from build123d import *

# Parameters (mm, degrees)
F2_DEPTH  = 3.175
F4_DEPTH  = 3.175
F5_R      = 0.8001
F6_DEPTH  = 3.2004
F7_R      = 0.8001
F8_DEPTH  = 25.4
F9_W      = 5.7083697757
F9_H      = 1.5914540656
F10_DEPTH = 3.175
F12_DEPTH = 25.4
F13_R     = 0.3937
F14_DEPTH = 25.4


with BuildPart() as f2:
    # F1 (on face) → F2 (new body)
    with BuildSketch(Plane.XY):
        with BuildLine():
            ThreePointArc((-1.5819782441, 9.3927083333), (-6.1504992572, -7.2730312723), (9.525, 0))
            ThreePointArc((9.525, 0), (7.2730312723, 6.1504992572), (1.5819782441, 9.3927083333))
            ThreePointArc((1.5819782441, 9.3927083333), (1.191708121, 9.4501564407), (0.7993940003, 9.4913958))
            ThreePointArc((0.7993940003, 9.4913958), (0, 8.7249), (-0.7993940003, 9.4913958))
            ThreePointArc((-0.7993940003, 9.4913958), (-1.191708121, 9.4501564407), (-1.5819782441, 9.3927083333))
        make_face()
        with BuildLine():
            ThreePointArc((0.7993940003, 9.4913958), (1.191708121, 9.4501564407), (1.5819782441, 9.3927083333))
            ThreePointArc((1.5819782441, 9.3927083333), (0, 11.1125), (-1.5819782441, 9.3927083333))
            ThreePointArc((-1.5819782441, 9.3927083333), (-1.191708121, 9.4501564407), (-0.7993940003, 9.4913958))
            ThreePointArc((-0.7993940003, 9.4913958), (-0.0168058077, 10.3249234806), (0.8001, 9.525))
            ThreePointArc((0.8001, 9.525), (0.7999234806, 9.5081941923), (0.7993940003, 9.4913958))
        make_face()
    extrude(amount=F2_DEPTH)

    # F3 (on Top) → F4 (join)
    with BuildSketch(Plane.XY):
        with BuildLine():
            ThreePointArc((0.7993940003, 9.4913958), (1.191708121, 9.4501564407), (1.5819782441, 9.3927083333))
            ThreePointArc((1.5819782441, 9.3927083333), (0, 11.1125), (-1.5819782441, 9.3927083333))
            ThreePointArc((-1.5819782441, 9.3927083333), (-1.191708121, 9.4501564407), (-0.7993940003, 9.4913958))
            ThreePointArc((-0.7993940003, 9.4913958), (-0.0168058077, 10.3249234806), (0.8001, 9.525))
            ThreePointArc((0.8001, 9.525), (0.7999234806, 9.5081941923), (0.7993940003, 9.4913958))
        make_face()
        with BuildLine():
            ThreePointArc((-0.7993940003, 9.4913958), (0, 9.525), (0.7993940003, 9.4913958))
            ThreePointArc((0.7993940003, 9.4913958), (0.7999234806, 9.5081941923), (0.8001, 9.525))
            ThreePointArc((0.8001, 9.525), (-0.0168058077, 10.3249234806), (-0.7993940003, 9.4913958))
        make_face()
        with BuildLine():
            ThreePointArc((4.2410481532, -8.5287241462), (6.5317636161, -8.99020135), (6.8007427217, -6.6689971835))
            ThreePointArc((6.8007427217, -6.6689971835), (6.51877471, -6.9448687015), (6.2256258064, -7.2088284984))
            ThreePointArc((6.2256258064, -7.2088284984), (6.3542336867, -7.4427136488), (6.3987545281, -7.7058868714))
            ThreePointArc((6.3987545281, -7.7058868714), (5.8298612048, -8.4718525904), (4.9321791435, -8.1485725067))
            ThreePointArc((4.9321791435, -8.1485725067), (4.5905504655, -8.3458056186), (4.2410481532, -8.5287241462))
        make_face()
        with BuildLine():
            ThreePointArc((4.9321791435, -8.1485725067), (5.5986545281, -7.7058868714), (6.2256258064, -7.2088284984))
            ThreePointArc((6.2256258064, -7.2088284984), (5.1283675477, -7.0585923742), (4.9321791435, -8.1485725067))
        make_face()
        with BuildLine():
            ThreePointArc((9.4218546282, 1.3979557805), (10.5686155373, 3.43395135), (8.4441383039, 4.4070572159))
            ThreePointArc((8.4441383039, 4.4070572159), (8.6193748012, 4.0536407137), (8.779827493, 3.6932714756))
            ThreePointArc((8.779827493, 3.6932714756), (9.5154003585, 3.6004167674), (9.8589133177, 2.9433868714))
            ThreePointArc((9.8589133177, 2.9433868714), (9.6960868018, 2.4596074625), (9.2738801556, 2.1727337295))
            ThreePointArc((9.2738801556, 2.1727337295), (9.3558909247, 1.7868771657), (9.4218546282, 1.3979557805))
        make_face()
        with BuildLine():
            ThreePointArc((9.2738801556, 2.1727337295), (9.0588133177, 2.9433868714), (8.779827493, 3.6932714756))
            ThreePointArc((8.779827493, 3.6932714756), (8.297872999, 2.6961423742), (9.2738801556, 2.1727337295))
        make_face()
        with BuildLine():
            ThreePointArc((-8.2587133177, 2.9433868714), (-8.4017834218, 3.3999739122), (-8.779827493, 3.6932714756))
            ThreePointArc((-8.779827493, 3.6932714756), (-9.0588133177, 2.9433868714), (-9.2738801556, 2.1727337295))
            ThreePointArc((-9.2738801556, 2.1727337295), (-8.5750339088, 2.3061133873), (-8.2587133177, 2.9433868714))
        make_face()
        with BuildLine():
            ThreePointArc((-6.2256258064, -7.2088284984), (-6.51877471, -6.9448687015), (-6.8007427217, -6.6689971835))
            ThreePointArc((-6.8007427217, -6.6689971835), (-6.5317636161, -8.99020135), (-4.2410481532, -8.5287241462))
            ThreePointArc((-4.2410481532, -8.5287241462), (-4.5905504655, -8.3458056186), (-4.9321791435, -8.1485725067))
            ThreePointArc((-4.9321791435, -8.1485725067), (-6.0689415084, -8.3531813686), (-6.2256258064, -7.2088284984))
        make_face()
        with BuildLine():
            ThreePointArc((-4.7985545281, -7.7058868714), (-5.3354813054, -6.9503077128), (-6.2256258064, -7.2088284984))
            ThreePointArc((-6.2256258064, -7.2088284984), (-5.5986545281, -7.7058868714), (-4.9321791435, -8.1485725067))
            ThreePointArc((-4.9321791435, -8.1485725067), (-4.8326888091, -7.9370935482), (-4.7985545281, -7.7058868714))
        make_face()
        with BuildLine():
            ThreePointArc((-0.7993940003, 9.4913958), (0, 8.7249), (0.7993940003, 9.4913958))
            ThreePointArc((0.7993940003, 9.4913958), (0, 9.525), (-0.7993940003, 9.4913958))
        make_face()
        with BuildLine():
            ThreePointArc((6.3987545281, -7.7058868714), (6.3542336867, -7.4427136488), (6.2256258064, -7.2088284984))
            ThreePointArc((6.2256258064, -7.2088284984), (5.5986545281, -7.7058868714), (4.9321791435, -8.1485725067))
            ThreePointArc((4.9321791435, -8.1485725067), (5.8298612048, -8.4718525904), (6.3987545281, -7.7058868714))
        make_face()
        with BuildLine():
            ThreePointArc((9.8589133177, 2.9433868714), (9.5154003585, 3.6004167674), (8.779827493, 3.6932714756))
            ThreePointArc((8.779827493, 3.6932714756), (9.0588133177, 2.9433868714), (9.2738801556, 2.1727337295))
            ThreePointArc((9.2738801556, 2.1727337295), (9.6960868018, 2.4596074625), (9.8589133177, 2.9433868714))
        make_face()
        with BuildLine():
            ThreePointArc((-9.2738801556, 2.1727337295), (-9.0588133177, 2.9433868714), (-8.779827493, 3.6932714756))
            ThreePointArc((-8.779827493, 3.6932714756), (-9.8197536364, 3.1906313686), (-9.2738801556, 2.1727337295))
        make_face()
        with BuildLine():
            ThreePointArc((-4.9321791435, -8.1485725067), (-5.5986545281, -7.7058868714), (-6.2256258064, -7.2088284984))
            ThreePointArc((-6.2256258064, -7.2088284984), (-6.0689415084, -8.3531813686), (-4.9321791435, -8.1485725067))
        make_face()
        with BuildLine():
            ThreePointArc((-8.779827493, 3.6932714756), (-8.6193748012, 4.0536407137), (-8.4441383039, 4.4070572159))
            ThreePointArc((-8.4441383039, 4.4070572159), (-10.5686155373, 3.43395135), (-9.4218546282, 1.3979557805))
            ThreePointArc((-9.4218546282, 1.3979557805), (-9.3558909247, 1.7868771657), (-9.2738801556, 2.1727337295))
            ThreePointArc((-9.2738801556, 2.1727337295), (-9.8197536364, 3.1906313686), (-8.779827493, 3.6932714756))
        make_face()
    extrude(amount=F4_DEPTH)

    # F5 (on face) → F6 (cut)
    with BuildSketch(Plane.XY.offset(3.175)):
        with Locations((0, 9.525)):
            Circle(F5_R)
        with Locations((-9.0588133177, 2.9433868714)):
            Circle(F5_R)
        with Locations((-5.5986545281, -7.7058868714)):
            Circle(F5_R)
        with Locations((5.5986545281, -7.7058868714)):
            Circle(F5_R)
        with Locations((9.0588133177, 2.9433868714)):
            Circle(F5_R)
    extrude(amount=-F6_DEPTH, mode=Mode.SUBTRACT)

    # F7 (on face) → F8 (cut)
    with BuildSketch(Plane.XY.offset(3.175)):
        with BuildLine():
            ThreePointArc((6.8007427217, -6.6689971835), (8.8176725791, -3.6019821332), (9.525, 0))
            Line((9.525, 0), (0, 0))
            Line((0, 0), (0, -9.525))
            ThreePointArc((0, -9.525), (2.1782478632, -9.2725865456), (4.2410481532, -8.5287241462))
            ThreePointArc((4.2410481532, -8.5287241462), (6.5317636161, -8.99020135), (6.8007427217, -6.6689971835))
        make_face()
        with Locations((5.5986545281, -7.7058868714)):
            Circle(F7_R, mode=Mode.SUBTRACT)
    extrude(amount=-F8_DEPTH, mode=Mode.SUBTRACT)

    # F9 (on face) → F10 (join)
    with BuildSketch(Plane.XY.offset(3.175)):
        with Locations((4.8052559723, 0.7957270328)):
            Rectangle(F9_W, F9_H)
    extrude(amount=F10_DEPTH)

    # F11 (on face) → F12 (cut)
    with BuildSketch(Plane.XZ):
        with BuildLine():
            Line((1.9510710845, 6.35), (1.9510710845, 4.7498))
            ThreePointArc((1.9510710845, 4.7498), (2.4197588132, 5.8813122713), (3.5512710845, 6.35))
            Line((3.5512710845, 6.35), (1.9510710845, 6.35))
        make_face()
        with BuildLine():
            Line((7.6594408602, 6.35), (6.0592408602, 6.35))
            ThreePointArc((6.0592408602, 6.35), (7.1907531314, 5.8813122713), (7.6594408602, 4.7498))
            Line((7.6594408602, 4.7498), (7.6594408602, 6.35))
        make_face()
    extrude(amount=-F12_DEPTH, mode=Mode.SUBTRACT)

    # F13 (on face) → F14 (cut)
    with BuildSketch(Plane.XZ):
        with Locations((6.645900663, 5.5013904348)):
            Circle(F13_R)
        with Locations((2.9646112816, 5.5013904348)):
            Circle(F13_R)
    extrude(amount=-F14_DEPTH, mode=Mode.SUBTRACT)


solid = f2.part
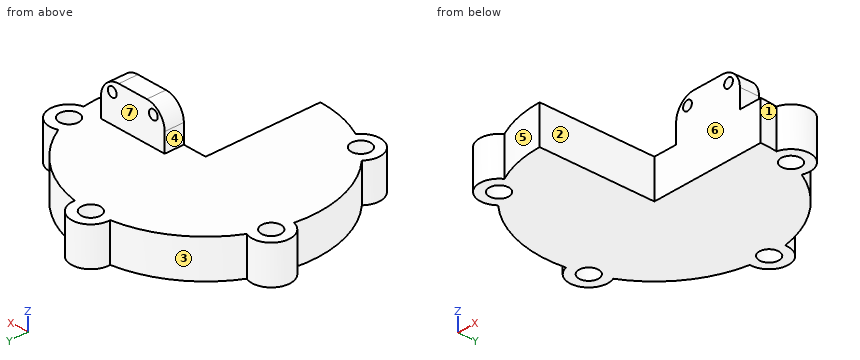
Design review of the part built by this model. Coordinates are the model's own, in mm. Face numbers are marked on the shaded views. A direction names the side the tool comes from. Give positions to 0.01 mm unless a question says otherwise; leave off trailing zeros. Loops run counter-clockwise (first coordinate to the right, second up) from the corner with the lowest first, then second, coordinate; pieces in that order, holes last. Notation, with made-up numbers: M -30,46 L 18,46 A37 ccw 18,85 Z; hole C 70,-33.75 d9. An arc over 180 degrees is marked long. Answer as a JSON object with one key per item and string values.
Item 1: Wall thickness on line 1 along X through (y, z) = (9.5, 1.25); line 2 along Z through (x, y) = (-3.75, 0.75) (3 decimals); line 3 along Y through (x, z) = (7, 4.5): over which ranges is each line inside the solid? List them lowest first.
Output values:
{"line 1": "x = -1.59 to -0.8, 0.8 to 1.59", "line 2": "z = 0 to 3.175", "line 3": "y = 0 to 1.59"}
Item 2: We need section B-B (z = 1.75). Count the separate pieces of the cut face and the enclosed holes in it, and give its area (3 significant figures).
Output values:
{"separate pieces": "1", "enclosed holes": "4", "area": "222 mm2"}
Item 3: We need section C-C (x = 4.5). State the section outline as (y, z) points (3 decimals), and give its area (3 significant figures).
Output values:
{"outline": "M 0,0 L 8.395,0 L 8.395,3.175 L 1.591,3.175 L 1.591,6.35 L 0,6.35 Z", "area": "31.7 mm2"}
Item 4: We need section D-D (z = 4.25). State the section outline as (x, y) points, and give its area (3 significant figures).
Output values:
{"outline": "M 1.95,0 L 7.66,0 L 7.66,1.59 L 1.95,1.59 Z", "area": "9.08 mm2"}
Item 5: Machinability: for the marked faces 4, 5, 6 and 7, which of the approach directions +Z, -Z, +X, -X, +Y, -Y give a long, thin tool a straight path to every point of the face, cutting with its end or side? Answer none if there is none.
Output values:
{"face 4": "+Z, -X, +Y, -Y", "face 5": "+Z, -Z, -Y", "face 6": "+Z, -Z, +X, -Y", "face 7": "+Z, +X, -X, +Y"}
Item 6: Mouldability with a two-part tool opening along Y and no side actions: class the marked faces 1, 2 and 3 as pulls with the +Y half, pulls with the -Y half, needs draft (parallel to the pull), parting line crosses it, or undercut.
Output values:
{"face 1": "undercut", "face 2": "needs draft", "face 3": "pulls with the +Y half"}
Item 7: For P1, Ø1.5, axis at x = -1, z = 3, coming from the +Y side; P2, Ø2.5, axis at x = 5, z = 5, coming from the +Y side; P3, Ø0.5, axis at y = 1, z = 4, coming from the +X side; P4, Ø1.5, axis at x = -6.5, z = 4, coming from the -Y side, all flat-tipped, find the tip position at first contact; note any pin that passes through.
Output values:
{"P1": "stops at y = 11.09", "P2": "stops at y = 1.59", "P3": "stops at x = 7.66", "P4": "passes through"}
Item 8: We need section A-A (y = 1). State the section outline as (x, z) points (3 decimals).
Output values:
{"outline": "M -9.472,0 L 9.472,0 L 9.472,3.175 L 7.659,3.175 L 7.659,4.75 A1.6 ccw 6.059,6.35 L 3.551,6.35 A1.6 ccw 1.951,4.75 L 1.951,3.175 L -9.472,3.175 Z; hole C 2.965,5.501 d0.787; hole C 6.646,5.501 d0.787"}
